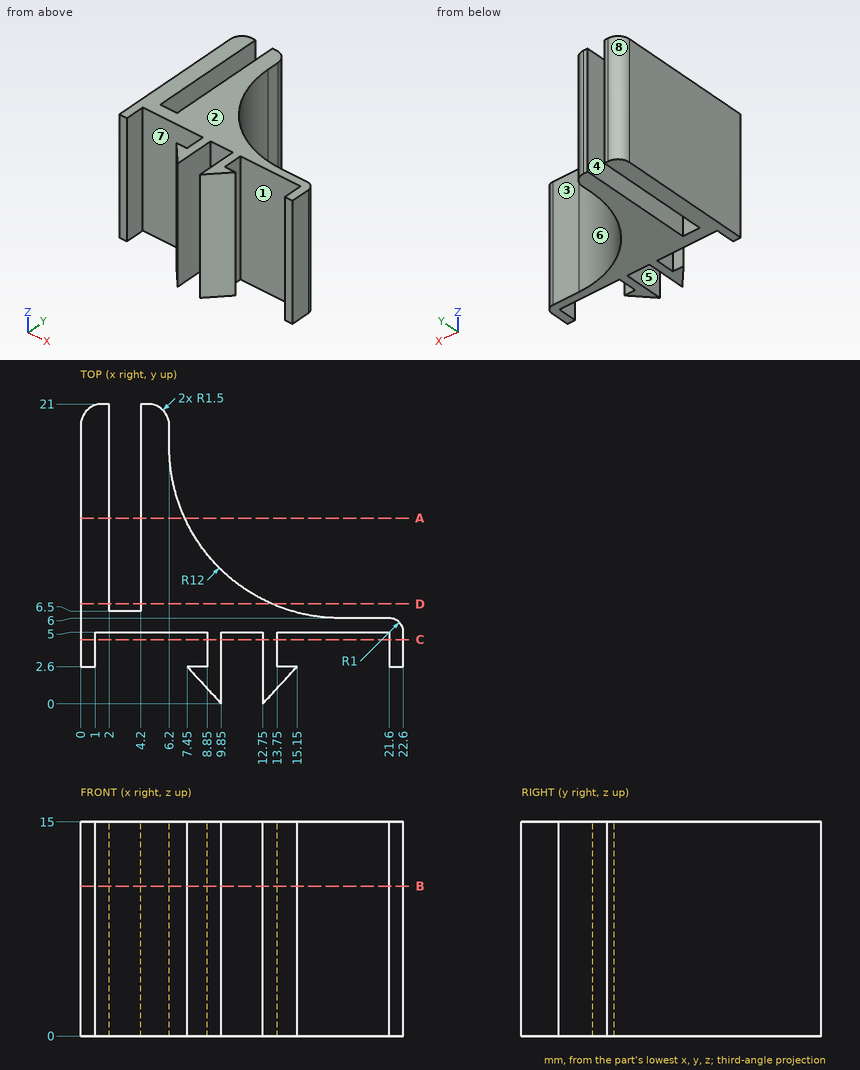
Job drawing, mm, ordinate dimensions from the low corner. One solid piece. A direction names the side the tool comes from. Give positions to 0.01 mm unless a question says otherwise; leave off trailing zeros. Write each loop counter-clockwise with the first axis right and the second up, starting at its lowest first coordinate (ties: lowest second). Pieces come first, ordered by that corner, then holes. Notation, with made-up numbers: (-15, 25) - (10, 25) arc R20 cw to (10, 43) - close; hole circle Ø5 at (-0.75, -24). An arc over 180 degrees is marked (long way). Answer as CSV lines item,"result".
1. Band-saw the part on C-C (y = 4.5). Write the cut outline in (x, z).
Responses:
outline,"(0, 0) - (1, 0) - (1, 15) - (0, 15) - close; (8.85, 0) - (9.85, 0) - (9.85, 15) - (8.85, 15) - close; (12.75, 0) - (13.75, 0) - (13.75, 15) - (12.75, 15) - close; (21.6, 0) - (22.6, 0) - (22.6, 15) - (21.6, 15) - close"
2. Band-saw the part on D-D (y = 7). Write the cut outline in (x, z), and give its area (3 significant figures).
Responses:
outline,"(0, 0) - (2, 0) - (2, 15) - (0, 15) - close; (4.2, 0) - (13.4, 0) - (13.4, 15) - (4.2, 15) - close"
area,"168 mm2"
3. Two-plate mould, pull along X, no slides. Class the marked faces 6, 7 and 8: +X half, -X half, draft (parallel to the pull), parting line (faces both ways), or undercut.
Responses:
face 6,"+X half"
face 7,"undercut"
face 8,"-X half"
4. Pin check, flat tips, straight feed: pin 1 (0.7 mm diameter, centred on x = 8.5, z = 7.5, fed in from +Y); pin 2 (4 mm diameter, centred on x = 6.5, z = 6.5, fed in from -Y); pin 3 (2 mm diameter, centred on y = 9, z = 9, fed in from -X); pin 4 (1.5 mm diameter, centred on y = 13, z = 9.5, fed in from +X). Stop position of each tip, or through.
Responses:
pin 1,"stops at y = 11.44"
pin 2,"stops at y = 1.46"
pin 3,"stops at x = 0"
pin 4,"stops at x = 7.67"
5. Band-saw the part on A-A (y = 13). Write the cut outline in (x, z), and give its area (3 significant figures).
Responses:
outline,"(0, 0) - (2, 0) - (2, 15) - (0, 15) - close; (4.2, 0) - (7.29, 0) - (7.29, 15) - (4.2, 15) - close"
area,"76.4 mm2"
6. 3-axis set-ups, long thin cutter, end or side, ignore diameter. For the marked faces 1, 2, 3, 4 and 5: which of +Z, -Z, +X, -X, +Y, -Y reach the whole face in a straight line?
Responses:
face 1,"+Z, -Z"
face 2,"+Z, +X, -X, +Y, -Y"
face 3,"+Z, -Z, +X, +Y"
face 4,"+Z, -Z, +Y"
face 5,"+Z, -Z, -Y"
7. Band-saw the part on B-B (z = 10.5). Write the cut outline in (x, y).
Responses:
outline,"(0, 2.6) - (1, 2.6) - (1, 5) - (8.85, 5) - (8.85, 2.6) - (7.45, 2.6) - (9.85, 0) - (9.85, 5) - (12.75, 5) - (12.75, 0) - (15.15, 2.6) - (13.75, 2.6) - (13.75, 5) - (21.6, 5) - (21.6, 2.6) - (22.6, 2.6) - (22.6, 5) arc R1 ccw to (21.6, 6) - (18.2, 6) arc R12 cw to (6.2, 18) - (6.2, 19.5) arc R1.5 ccw to (4.7, 21) - (4.2, 21) - (4.2, 6.5) - (2, 6.5) - (2, 21) - (1.5, 21) arc R1.5 ccw to (0, 19.5) - close"
8. Drill centre lines: L1, parallel to X at y = 4, z = 12.25; L2, parallel to X at y = 19.25, z = 8; L3, parallel to Y at x = 3.25, z = 3.5. Where is each one in solid material? Low to high. Write a range as [from, to].
Responses:
L1,"x = [0, 1], [8.85, 9.85], [12.75, 13.75], [21.6, 22.6]"
L2,"x = [0, 2], [4.2, 6.2]"
L3,"y = [5, 6.5]"
